```python
from build123d import *

# Parameters (mm, degrees)
BOSS_EXTRUDE1_DEPTH = 19.05
SKETCH2_W           = 19.08812797
SKETCH2_H           = 1.877723278
BOSS_EXTRUDE3_DEPTH = 25.4
SKETCH3_R           = 9.544063985
BOSS_EXTRUDE4_DEPTH = 19.08812797


with BuildPart() as part:
    # Sketch1 → Boss-Extrude1 (new body)
    with BuildSketch(Plane.XY):
        Polygon((-33.631481481, 34.502858519), (-33.631481481, -34.502858519), (33.631481481, -34.502858519), (33.631481481, 34.502858519), (6.35, 34.502858519), (6.35, 22.529183691), (31.75, 22.529183691), (31.75, -15.570816309), (-31.75, -15.570816309), (-31.75, 22.529183691), (-6.35, 22.529183691), (-6.35, 34.502858519), align=None)
    extrude(amount=BOSS_EXTRUDE1_DEPTH)

    # Sketch2 → Boss-Extrude3 (add)
    with BuildSketch(Plane.XZ.offset(34.502858519)):
        with Locations((0, 0.938861639)):
            Rectangle(SKETCH2_W, SKETCH2_H)
    extrude(amount=BOSS_EXTRUDE3_DEPTH)

    # Sketch3 → Boss-Extrude4 (add)
    with BuildSketch(Plane(origin=(0, 0, 0), x_dir=(-1, 0, 0), z_dir=(0, 0, -1))):
        with Locations((0, -59.902858519)):
            Circle(SKETCH3_R)
    extrude(amount=-BOSS_EXTRUDE4_DEPTH)


solid = part.part
```
Verification items for the finished model (mm, model axes). A direction names the side the tool comes from. Give positions to 0.01 mm unless a question says otherwise; leave off trailing zeros. Loops run counter-clockwise (first coordinate to the right, second up) from the corner with the lowest first, then second, coordinate; pieces in that order, holes last. Notation, with made-up numbers: M 3,31.5 L 15,31.5 A32 ccw 15,58.5 Z; hole C -9,64 d10. An arc over 180 degrees is marked long. One line per question, with ' | ' between items.
Item 1: Section check A-A, the plane z = 10.75. Record the cut outline in (x, y).
Completed:
outline: M -33.63,-34.5 L 33.63,-34.5 L 33.63,34.5 L 6.35,34.5 L 6.35,22.53 L 31.75,22.53 L 31.75,-15.57 L -31.75,-15.57 L -31.75,22.53 L -6.35,22.53 L -6.35,34.5 L -33.63,34.5 Z; C 0,-59.9 d19.09
Item 2: Draft check along X on faces 3 (the face through (2.07, -69.22, 9.41)), 4 (the face through (0, -60, 19.088)), 5 (the face through (-33.631, 0, 9)), 6 (the face through (0, -15.571, 9)). Enter one of: +X half, -X half, draft (parallel to the pull), parting line (faces both ways), or undercut.
Completed:
face 3: parting line | face 4: draft | face 5: -X half | face 6: undercut
Item 3: Section check D-D, the plane x = 0. Record the cut outline in (y, z).
Completed:
outline: M -69.45,0 L -15.57,0 L -15.57,19.05 L -34.5,19.05 L -34.5,1.88 L -50.36,1.88 L -50.36,19.09 L -69.45,19.09 Z
Item 4: Thickness scan on line 1 (Y direction, x = 26.5, z = 13); line 2 (X direction, y = 9, z = 9.5); line 3 (Y direction, x = 7.5, z = 17.5). Record the ranges inside material, lowest first. Write a range as [from, to].
Completed:
line 1: y = [-34.5, -15.57], [22.53, 34.5] | line 2: x = [-33.63, -31.75], [31.75, 33.63] | line 3: y = [-65.81, -54], [-34.5, -15.57], [22.53, 34.5]
Item 5: Section check C-C, the plane x = 8.5. Record the cut outline in (y, z).
Completed:
outline: M -64.24,0 L -15.57,0 L -15.57,19.05 L -34.5,19.05 L -34.5,1.88 L -55.56,1.88 L -55.56,19.09 L -64.24,19.09 Z; M 22.53,0 L 34.5,0 L 34.5,19.05 L 22.53,19.05 Z
Item 6: Depth check by flat-ended pin: P1, Ø0.6, axis at y = -44, z = 1, coming from the -X side; P2, Ø5.5, axis at x = 22, z = 11.5, coming from the -Y side; P3, Ø1, axis at x = -5, z = 6.5, coming from the +Y side. Enter the tip coordinate at first touch or a pass-through.
Completed:
P1: stops at x = -9.54 | P2: stops at y = -34.5 | P3: stops at y = -15.57
Item 7: Section check B-B, the plane y = 7. Record the cut outline in (x, z).
Completed:
outline: M -33.63,0 L -31.75,0 L -31.75,19.05 L -33.63,19.05 Z; M 31.75,0 L 33.63,0 L 33.63,19.05 L 31.75,19.05 Z
Item 8: Tool access check on faces 1 (the face through (-31.75, 3, 9)), 2 (the face through (6.35, 29, 9)). Record the directions out of +Z, -Z, +X, -X, +Y, -Y that give a thin tool (end or side, any length) a straight path to the whole face; none if there is none.
Completed:
face 1: +Z, -Z | face 2: +Z, -Z, +Y
